Part model, mm, in its own coordinate system. A direction names the side the tool comes from. Give positions to 0.01 mm unless a question says otherwise; leave off trailing zeros. Loops run counter-clockwise (first coordinate to the right, second up) from the corner with the lowest first, then second, coordinate; pieces in that order, holes last. Notation, with made-up numbers: M 80.25,71.5 L 136.25,71.5 A21 cw 136.25,102.5 Z; hole C 88.5,-19.75 d5. An arc over 180 degrees is marked long. Answer in a Markdown table with one row per item.
from build123d import *

# Parameters (mm, degrees)
SKETCH1_W           = 42.3
SKETCH1_H           = 42.3
BOSS_EXTRUDE1_DEPTH = 5
FILLET1_R           = 5
SKETCH2_R           = 1.75
CUT_EXTRUDE1_DEPTH  = 32.537992961
SKETCH3_R           = 11.25
CUT_EXTRUDE2_DEPTH  = 2
SKETCH4_R           = 9.5
CUT_EXTRUDE3_DEPTH  = 31.96199283
SKETCH5_R           = 3
CUT_EXTRUDE4_DEPTH  = 32.537992961
CIRPATTERN1_COUNT   = 6


with BuildPart() as part:
    # Sketch1 → Boss-Extrude1 (new, symmetric)
    with BuildSketch(Plane(origin=(0, 0, 0), x_dir=(1, 0, 0), z_dir=(0, 1, 0))):
        Rectangle(SKETCH1_W, SKETCH1_H)
    extrude(amount=BOSS_EXTRUDE1_DEPTH, both=True)

    # Fillet1
    fillet1_edges = [part.edges().sort_by_distance(p)[0] for p in [
        (21.15, 0, 21.15),
        (-21.15, 0, 21.15),
        (-21.15, 0, -21.15),
        (21.15, 0, -21.15),
    ]]
    fillet(fillet1_edges, radius=FILLET1_R)

    # Sketch2 → Cut-Extrude1 (cut, through all)
    with BuildSketch(Plane.XZ.offset(5)):
        with Locations(Location((-15.5, 15.5, 0), (0, 0, 270))):
            Circle(SKETCH2_R)
        with Locations(Location((15.5, 15.5, 0), (0, 0, 270))):
            Circle(SKETCH2_R)
        with Locations(Location((15.5, -15.5, 0), (0, 0, 270))):
            Circle(SKETCH2_R)
        with Locations(Location((-15.5, -15.5, 0), (0, 0, 270))):
            Circle(SKETCH2_R)
    extrude(amount=-CUT_EXTRUDE1_DEPTH, mode=Mode.SUBTRACT)

    # Sketch3 → Cut-Extrude2 (cut)
    with BuildSketch(Plane.XZ.offset(5)):
        with Locations(Location((0, 0, 0), (0, 0, 270))):
            Circle(SKETCH3_R)
    extrude(amount=-CUT_EXTRUDE2_DEPTH, mode=Mode.SUBTRACT)

    # Sketch4 → Cut-Extrude3 (cut, through all)
    with BuildSketch(Plane.XZ.offset(3)):
        with Locations(Location((0, 0, 0), (0, 0, 270))):
            Circle(SKETCH4_R)
    extrude(amount=-CUT_EXTRUDE3_DEPTH, mode=Mode.SUBTRACT)

    # Sketch5 → Cut-Extrude4 (cut, through all)
    with BuildSketch(Plane(origin=(0, 5, 0), x_dir=(1, 0, 0), z_dir=(0, 1, 0))):
        with Locations(Location((0, 14, 0), (0, 0, 270))):
            Circle(SKETCH5_R)
    cut_extrude4 = extrude(amount=-CUT_EXTRUDE4_DEPTH, mode=Mode.SUBTRACT)

    # CirPattern1: Cut-Extrude4 ×6 about axis
    cirpattern1_axis = Axis((0, 0, 0), (0, 1, 0))
    for i in range(1, CIRPATTERN1_COUNT):
        add(cut_extrude4.rotate(cirpattern1_axis, i * 360 / CIRPATTERN1_COUNT), mode=Mode.SUBTRACT)


solid = part.part
(1) Which spindle directions (+Z, -Z, +X, -X, +Y, -Y) get a long thin tool onto all of the face, cutting with end or side? Do faces 1 (the face through (-5.7, -4, -9.7)), 2 (the face through (0, 0, 21.15)). Say none if no direction does.
Recorded:
| item | result |
|---|---|
| face 1 | -Y |
| face 2 | +Z, +X, -X, +Y, -Y |
(2) Saw through at C-C (z = 15.5). Write the cut outline in (x, y).
Recorded:
| item | result |
|---|---|
| outline | M -21.15,-5 L -17.25,-5 L -17.25,5 L -21.15,5 Z; M -13.75,-5 L -2.6,-5 L -2.6,5 L -13.75,5 Z; M 2.6,-5 L 13.75,-5 L 13.75,5 L 2.6,5 Z; M 17.25,-5 L 21.15,-5 L 21.15,5 L 17.25,5 Z |
(3) Saw through at D-D (x = -12.5). Write the cut outline in (y, z).
Recorded:
| item | result |
|---|---|
| outline | M -5,-21.15 L 5,-21.15 L 5,-9.98 L -5,-9.98 Z; M -5,-4.02 L 5,-4.02 L 5,4.02 L -5,4.02 Z; M -5,9.98 L 5,9.98 L 5,21.15 L -5,21.15 Z |
(4) Saw through at B-B (x = -2.5). Write the cut outline in (y, z), plus the area to 3 significant figures.
Recorded:
| item | result |
|---|---|
| outline | M -5,-21.15 L 5,-21.15 L 5,-15.66 L -5,-15.66 Z; M -5,-12.34 L 5,-12.34 L 5,-9.17 L -3,-9.17 L -3,-10.97 L -5,-10.97 Z; M -5,10.97 L -3,10.97 L -3,9.17 L 5,9.17 L 5,12.34 L -5,12.34 Z; M -5,15.66 L 5,15.66 L 5,21.15 L -5,21.15 Z |
| area | 166 mm^2 |
(5) Pull direction Z, two halves, no side cores. Call faces 3 (the face through (-13.765, -0.07, -15.272)), 4 (the face through (-21.15, 0, 0)), 5 (the face through (-19.72, 0.07, 19.65)): +Z half, -Z half, draft (parallel to the pull), parting line (faces both ways), or undercut.
Recorded:
| item | result |
|---|---|
| face 3 | undercut |
| face 4 | draft |
| face 5 | +Z half |
(6) Drill centre lines: line 1 along X through (y, z) = (1.75, 0); line 2 along Z through (x, y) = (13.5, -1); line 3 along Z through (x, y) = (14, 0.25). Where is each one in solid material? Low to high.
Recorded:
| item | result |
|---|---|
| line 1 | x = -21.15 to -9.5, 9.5 to 21.15 |
| line 2 | z = -21.15 to -9.67, -4.33 to 4.33, 9.67 to 21.15 |
| line 3 | z = -21.15 to -16.4, -14.6 to -9.34, -4.66 to 4.66, 9.34 to 14.6, 16.4 to 21.15 |
(7) Saw through at A-A (z = 1.5). Write the cut outline in (x, y), plus the area to 3 significant figures.
Recorded:
| item | result |
|---|---|
| outline | M -21.15,-5 L -11.15,-5 L -11.15,-3 L -9.38,-3 L -9.38,5 L -21.15,5 Z; M 9.38,-3 L 11.15,-3 L 11.15,-5 L 21.15,-5 L 21.15,5 L 9.38,5 Z |
| area | 228 mm^2 |
